Work out the finished part from the listing and answer in its coordinate system (mm). Face numbers are marked on the shaded views. Give positions to 0.01 mm unless a question says otherwise; leave off trailing zeros. Loops run counter-clockwise (first coordinate to the right, second up) from the corner with the lowest first, then second, coordinate; pieces in that order, holes last.
from build123d import *

# Parameters (mm, degrees)
F0_W     = 83
F0_H     = 70
F1_DEPTH = 3
F2_R     = 15
F3_DEPTH = 10
F4_R     = 4
F5_DEPTH = 25


with BuildPart() as f1:
    # F0 (on Top) → F1 (new body)
    with BuildSketch(Plane.XY):
        Rectangle(F0_W, F0_H)
    extrude(amount=-F1_DEPTH)

    # F2 (on Front) → F3 (join, symmetric)
    with BuildSketch(Plane.XZ):
        with BuildLine():
            ThreePointArc((0, 0), (-11.667262, 4.832738), (-16.5, 16.5))
            Line((-16.5, 16.5), (-24.06125, 0))
            Line((-24.06125, 0), (0, 0))
        make_face()
        with BuildLine():
            Line((24.06125, 0), (16.5, 16.5))
            ThreePointArc((16.5, 16.5), (11.667262, 4.832738), (0, 0))
            Line((0, 0), (24.06125, 0))
        make_face()
        with BuildLine():
            ThreePointArc((0, 0), (11.667262, 4.832738), (16.5, 16.5))
            ThreePointArc((16.5, 16.5), (0, 33), (-16.5, 16.5))
            ThreePointArc((-16.5, 16.5), (-11.667262, 4.832738), (0, 0))
        make_face()
        with Locations((0, 16.5)):
            Circle(F2_R, mode=Mode.SUBTRACT)
    extrude(amount=F3_DEPTH, both=True)

    # F4 (on face) → F5 (cut)
    with BuildSketch(Plane(origin=(0, 0, -3), x_dir=(1, 0, 0), z_dir=(0, 0, -1))):
        with Locations((-27.5, -15)):
            Circle(F4_R)
        with Locations((-27.5, 15)):
            Circle(F4_R)
        with Locations((25.5, 15)):
            Circle(F4_R)
        with Locations((25.5, -15)):
            Circle(F4_R)
    extrude(amount=-F5_DEPTH, mode=Mode.SUBTRACT)


solid = f1.part
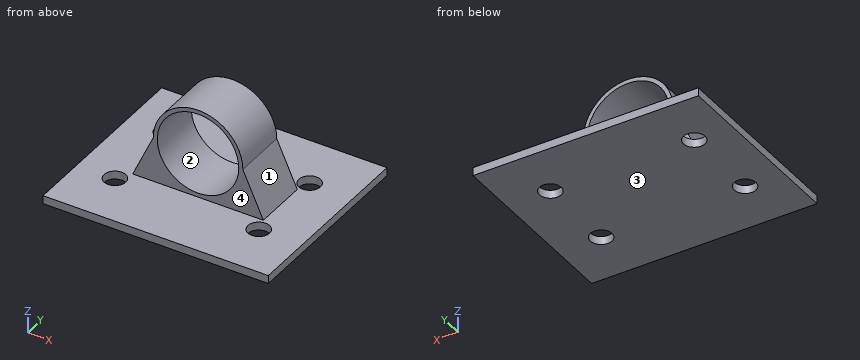
Item 1: Find section B-B, the plane y = -2. Write down the section's boundary in (x, z).
Item 2: Consider line 1 (X direction, y = 15, z = -2.4); line 2 (Y direction, x = -27.5, z = -1.7); line 3 (Z direction, x = 21.5, y = -18). Determine where each line is inside the solid, lowest interval first.
Item 3: Find section D-D, the plane y = -15. Write down the section's boundary in (x, z).
Item 4: Find section C-C, the plane x = 0. Write down the section's boundary in (y, z), plus the area to 3 significant figures.
Item 5: Flat-ended cylindrical pins translate along their axes: pin 1 Ø10.5 at (x, y) = (-27.5, -15) entering from +Z; pin 2 Ø8 at (x, z) = (7, 25.5) entering from +Y; pin 3 Ø16.5 at (x, z) = (0.5, 22.5) entering from +Y. Find the tip coordinate at first contact, or state that the pin passes through.
Item 6: Find section A-A, the plane x = -27.5. Write down the section's boundary in (y, z).
Item 7: Determine the mould class of the marked faces 1, 2, 3 and 4 for opening direction Z: released by +Z, released by -Z, zero draft, split by the parting line, or undercut.
Ans:
1. outline: (-41.5, -3) - (41.5, -3) - (41.5, 0) - (24.06, 0) - (16.5, 16.5) arc R16.5 ccw to (-16.5, 16.5) - (-24.06, 0) - (-41.5, 0) - close; hole circle Ø30 at (0, 16.5)
2. line 1: x = -41.5 to -31.5, -23.5 to 21.5, 29.5 to 41.5
2. line 2: y = -35 to -19, -11 to 11, 19 to 35
2. line 3: z = -3 to 0
3. outline: (-41.5, -3) - (-31.5, -3) - (-31.5, 0) - (-41.5, 0) - close; (-23.5, -3) - (21.5, -3) - (21.5, 0) - (-23.5, 0) - close; (29.5, -3) - (41.5, -3) - (41.5, 0) - (29.5, 0) - close
4. outline: (-35, -3) - (35, -3) - (35, 0) - (10, 0) - (10, 1.5) - (-10, 1.5) - (-10, 0) - (-35, 0) - close; (-10, 31.5) - (10, 31.5) - (10, 33) - (-10, 33) - close
4. area: 270 mm2
5. pin 1: stops at z = 0
5. pin 2: stops at y = 10
5. pin 3: passes through
6. outline: (-35, -3) - (-19, -3) - (-19, 0) - (-35, 0) - close; (-11, -3) - (11, -3) - (11, 0) - (-11, 0) - close; (19, -3) - (35, -3) - (35, 0) - (19, 0) - close
7. face 1: released by +Z
7. face 2: undercut
7. face 3: released by -Z
7. face 4: zero draft
